from build123d import *

# Parameters (mm, degrees)
F0_W     = 120
F0_H     = 120
F1_DEPTH = 25
F3_D     = 4.5
F4_R     = 53.34
F4_R_2   = 30.25
F5_DEPTH = 14.732
F6_R     = 6.35
F9_W     = 19.05
F9_H     = 15


with BuildPart() as f1:
    # F0 (on Top) → F1 (new body)
    with BuildSketch(Plane.XY):
        Rectangle(F0_W, F0_H)
    extrude(amount=-F1_DEPTH)

    # F3 (through all)
    with Locations(Plane.XY):
        with Locations((-52.5, -52.5), (52.5, -52.5), (52.5, 52.5), (-52.5, 52.5)):
            Hole(F3_D / 2)

    # F4 (on face) → F5 (cut)
    with BuildSketch(Plane.XY):
        Circle(F4_R)
        Circle(F4_R_2, mode=Mode.SUBTRACT)
    extrude(amount=-F5_DEPTH, mode=Mode.SUBTRACT)

    # F6
    f6_edges = [f1.edges().sort_by_distance(p)[0] for p in [
        (60, -60, -12.5),
        (-60, -60, -12.5),
        (60, 60, -12.5),
        (-60, 60, -12.5),
    ]]
    fillet(f6_edges, radius=F6_R)

    # F9 (on face) → F10 (revolve, cut)
    with BuildSketch(Plane(origin=(0, 0, 0), x_dir=(-0.7071067812, 0.7071067812, 0), z_dir=(0.7071067812, 0.7071067812, 0))):
        with Locations((-72.6975576213, -12.5)):
            Rectangle(F9_W, F9_H)
    revolve(axis=Axis((0, 0, 0), (0, 0, 1)), mode=Mode.SUBTRACT)


solid = f1.part
Here's how the part is built. I have some questions about the finished solid (model axes, mm). A direction names the side the tool comes from. Give positions to 0.01 mm unless a question says otherwise; leave off trailing zeros. Order: outer loops, then holes, each group sorted by start corner. A loop starts at its lowest first (then second) coordinate and runs counter-clockwise, first axis right, second up. Notation, with made-up numbers: (20, 44) -> (51, 44) arc R18 cw to (51, 54) -> close; hole circle Ø4 at (71, 36.5). An arc over 180 degrees is marked (long way). Use a Markdown table: item, result. Add a question column.
Item 1: Imagine slicing it at B-B on y = 0. Please give me the cut outline in (x, z).
Item 2: If we mould it in two halves opening along Z, with no side actions, what happens to faces 1 (the face through (-50.84, -50.98, -22.53)), 2 (the face through (-48, 48, -20)), 3 (the face through (-54, 1, 0)), 4 (the face through (44.38, -44.96, -12.4))? For each: pulls with the +Z half, pulls with the -Z half, needs draft (parallel to the pull), parting line crosses it, or undercut.
Item 3: Imagine slicing it at A-A on z = -1.75. Please give me the cut outline in (x, y).
Item 4: Imagine slicing it at D-D on y = 23. Please give me the cut outline in (x, z).
Item 5: For faces 5 (the face through (-58.19, -58.09, -22.54)), 6 (the face through (-44.96, -44.38, -12.4)), 7 (the face through (44.96, 44.38, -12.4)), which set-ups out of +Z, -Z, +X, -X, +Y, -Y let a thin tool reach every point of the face, with its end or its side?
Item 6: I need wall thicknesses on line 1 (Y direction, x = 52.5, z = -22.95); line 2 (Y direction, x = -11, z = -6.25); line 3 (X direction, y = 8, z = -7.5). Which ranges of each line are inside material? Lowest first, please.
Item 7: Will these pins go through, and if not, where does the flat tip stop? pin 1 (5 mm diameter, centred on x = -35, y = 35, fed in from +Z); pin 2 (3.5 mm diameter, centred on x = -52.5, y = -52.5, fed in from -Z); pin 3 (5 mm diameter, centred on y = 34.5, z = -15, fed in from +X); pin 4 (2 mm diameter, centred on y = 22, z = -16, fed in from -X).
Data:
| question | item | result |
|---|---|---|
| 1 | outline | (-60, -25) -> (60, -25) -> (60, 0) -> (53.34, 0) -> (53.34, -14.73) -> (30.25, -14.73) -> (30.25, 0) -> (-30.25, 0) -> (-30.25, -14.73) -> (-53.34, -14.73) -> (-53.34, 0) -> (-60, 0) -> close |
| 2 | face 1 | needs draft |
| 2 | face 2 | undercut |
| 2 | face 3 | pulls with the +Z half |
| 2 | face 4 | undercut |
| 3 | outline | (-60, -53.65) arc R6.35 ccw to (-53.65, -60) -> (53.65, -60) arc R6.35 ccw to (60, -53.65) -> (60, 53.65) arc R6.35 ccw to (53.65, 60) -> (-53.65, 60) arc R6.35 ccw to (-60, 53.65) -> close; circle Ø60.5 at (0, 0); hole circle Ø4.5 at (-52.5, -52.5); hole circle Ø4.5 at (-52.5, 52.5); hole circle Ø106.68 at (0, 0); hole circle Ø4.5 at (52.5, -52.5); hole circle Ø4.5 at (52.5, 52.5) |
| 4 | outline | (-60, -25) -> (60, -25) -> (60, -20) -> (58.84, -20) -> (58.84, -5) -> (60, -5) -> (60, 0) -> (48.13, 0) -> (48.13, -14.73) -> (19.65, -14.73) -> (19.65, 0) -> (-19.65, 0) -> (-19.65, -14.73) -> (-48.13, -14.73) -> (-48.13, 0) -> (-60, 0) -> (-60, -5) -> (-58.84, -5) -> (-58.84, -20) -> (-60, -20) -> close |
| 5 | face 5 | +Z, -Z, -X, -Y |
| 5 | face 6 | -X, -Y |
| 5 | face 7 | +X, +Y |
| 6 | line 1 | y = -60 to -54.75, -50.25 to 50.25, 54.75 to 60 |
| 6 | line 2 | y = -60 to -52.19, -28.18 to 28.18, 52.19 to 60 |
| 6 | line 3 | x = -60 to -52.74, -29.17 to 29.17, 52.74 to 60 |
| 7 | pin 1 | stops at z = -14.73 |
| 7 | pin 2 | passes through |
| 7 | pin 3 | stops at x = 54.47 |
| 7 | pin 4 | stops at x = -59.58 |
